The figure shows three views and two pictorial views of one solid part (mm, origin at its lowest corner). Answer the questions. Coordinates: 2 decimals unless noted, no trailing zeros. Order: outer loops, then holes, each group sorted by start corner. A loop starts at its lowest first (then second) coordinate and runs counter-clockwise, first axis right, second up. Notation, with made-up numbers: (81.5, -25.75) - (131.5, -25.75) arc R11 cw to (131.5, -12.75) - close; hole circle Ø2 at (67.5, 51). An arc over 180 degrees is marked (long way). Answer as a JSON object with one key per item and string values. Group by question number.
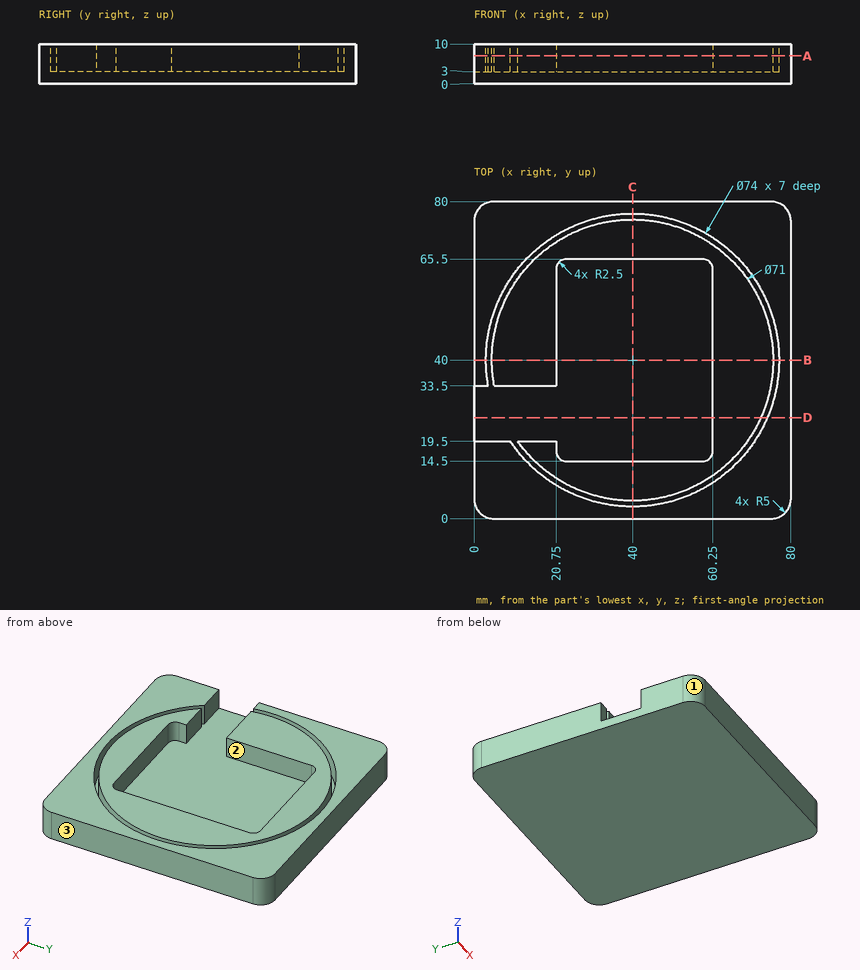
1. For a pull along Y with two mould halves and no side action, classify the marked faces 1, 2 and 3 as pulls with the +Y half, pulls with the -Y half, needs draft (parallel to the pull), parting line crosses it, or undercut.
2. Straight lines are drawn through the part: L1, parallel to Y at x = 40.5, z = 9; L2, parallel to X at y = 40, z = 6.5; L3, parallel to Y at x = 34.5, z = 7.5. For each, find the intervals that lie inside material, in ascending order.
3. Given pin 1 (8 mm diameter, centred on x = 15, y = 13, fed in from +Z); pin 2 (1.8 mm diameter, centred on x = 2, z = 6, fed in from -Y), each flat-ended and moving along its own axis, determine where each tip first touches the part or whether it passes through.
4. A cutting plane is placed at B-B on y = 40. Write down the section's boundary in (x, z), and give its area (4 significant figures).
5. A cutting plane is placed at C-C on x = 40. Write down the section's boundary in (y, z).
6. A cutting plane is placed at D-D on y = 25.5. Write down the section's boundary in (x, z).
7. A cutting plane is placed at A-A on z = 7. Write down the section's boundary in (x, y), and give its area (3 significant figures).
Derived:
{
 "1": {"face 1": "pulls with the -Y half", "face 2": "undercut", "face 3": "needs draft"},
 "2": {"L1": "y = 0 to 3, 4.5 to 14.5, 65.5 to 75.5, 77 to 80", "L2": "x = 0 to 3, 4.5 to 20.75, 60.25 to 75.5, 77 to 80", "L3": "y = 0 to 3.41, 4.93 to 14.5, 65.5 to 75.07, 76.59 to 80"},
 "3": {"pin 1": "stops at z = 10", "pin 2": "stops at y = 0.46"},
 "4": {"outline": "(0, 0) - (80, 0) - (80, 10) - (77, 10) - (77, 3) - (75.5, 3) - (75.5, 10) - (60.25, 10) - (60.25, 3) - (20.75, 3) - (20.75, 10) - (4.5, 10) - (4.5, 3) - (3, 3) - (3, 10) - (0, 10) - close", "area": "502.5 mm2"},
 "5": {"outline": "(0, 0) - (80, 0) - (80, 10) - (77, 10) - (77, 3) - (75.5, 3) - (75.5, 10) - (65.5, 10) - (65.5, 3) - (14.5, 3) - (14.5, 10) - (4.5, 10) - (4.5, 3) - (3, 3) - (3, 10) - (0, 10) - close"},
 "6": {"outline": "(0, 0) - (80, 0) - (80, 10) - (74.04, 10) - (74.04, 3) - (72.4, 3) - (72.4, 10) - (60.25, 10) - (60.25, 3) - (0, 3) - close"},
 "7": {"outline": "(0, 5) arc R5 ccw to (5, 0) - (75, 0) arc R5 ccw to (80, 5) - (80, 75) arc R5 ccw to (75, 80) - (5, 80) arc R5 ccw to (0, 75) - (0, 33.5) - (3.58, 33.5) arc R37 cw (long way) to (9.2, 19.5) - (0, 19.5) - close; (5.1, 33.5) - (20.75, 33.5) - (20.75, 63) arc R2.5 cw to (23.25, 65.5) - (57.75, 65.5) arc R2.5 cw to (60.25, 63) - (60.25, 17) arc R2.5 cw to (57.75, 14.5) - (23.25, 14.5) arc R2.5 cw to (20.75, 17) - (20.75, 19.5) - (11.02, 19.5) arc R35.5 ccw (long way) to start", "area": "3,760 mm2"}
}
